Check sheet for the modelled part. Datum: model origin and axes. Units: mm. A direction names the side the tool comes from. Round coordinates to 2 decimals unless told otherwise and drop trailing zeros. Write each loop counter-clockwise with the first axis right and the second up, starting at its lowest first coordinate (ties: lowest second). Pieces come first, ordered by that corner, then holes. Notation, with made-up numbers: (30.5, -35.5) - (79.5, -35.5) arc R30 cw to (79.5, -8.5) - close; hole circle Ø3 at (83, 39.25). An arc over 180 degrees is marked (long way). Answer as a JSON object with one key per item and string values. Group by question number.
Item 1: Thickness scan on line 1 (Z direction, x = -5.25, y = 4) (3 decimals); line 2 (Y direction, x = 1.5, z = -66.5); line 3 (Y direction, x = 0.25, z = -3.5). Record the ranges inside material, lowest first.
Item 2: Sectioned sample at B-B on z = 7.5. Record the boundary of the cut face in (x, y) (3 decimals), plus the area to 3 significant figures.
Item 3: Release check for a two-part mould opening along Z. For faces 1 (the flat face through (2, -3, -53.975)), 2 (the flat face through (0.1, 3.4, 63.5)), 3 (the flat face through (5.657, -6.238, 61.89)) record: pulls with the +Z half, pulls with the -Z half, needs draft (parallel to the pull), parting line crosses it, or undercut.
Item 4: Set-up check for faces 4 (the cylindrical face through (-0.69, -3.1, -69.94)), 5 (the cylindrical face through (6.194, 0.039, 61.89)), 6 (the cylindrical face through (-3.78, -2.9, 57.43)): record each of +Z, -Z, +X, -X, +Y, -Y from which the full face is reachable in a straight line by a thin tool's end or side.
Item 5: Gauge pin test, flat ends, axial feed: P1, Ø1.5, axis at x = -2.5, y = -10.5, coming from the +Z side; P2, Ø4, axis at x = 3, z = -51.5, coming from the +Y side; P3, Ø6, axis at y = -5.5, z = -44, coming from the -X side. Record the tip position at first contact, or that the pin passes through.
```python
from build123d import *

# Parameters (mm, degrees)
SKETCH1_R           = 3.175
BOSS_EXTRUDE1_DEPTH = 53.975
SKETCH2_R           = 4.7625
BOSS_EXTRUDE2_DEPTH = 6.35
BOSS_EXTRUDE3_DEPTH = 3.175
FILLET1_R           = 0.635
BOSS_EXTRUDE4_START = 12.7
SKETCH4_R           = 3.175
BOSS_EXTRUDE4_DEPTH = 12.7


with BuildPart() as part:
    # Sketch1 → Boss-Extrude1 (new body)
    with BuildSketch(Plane.XY):
        Circle(SKETCH1_R)
    boss_extrude1 = extrude(amount=BOSS_EXTRUDE1_DEPTH)

    # Sketch2 → Boss-Extrude2 (add)
    with BuildSketch(Plane.XY.offset(53.975)):
        Circle(SKETCH2_R)
    boss_extrude2 = extrude(amount=BOSS_EXTRUDE2_DEPTH)

    # Sketch3 → Boss-Extrude3 (add)
    with BuildSketch(Plane.XY.offset(60.325)):
        with BuildLine():
            Line((-0.215682611, 14.2875), (0.215682611, 14.2875))
            ThreePointArc((0.215682611, 14.2875), (3.60364364, 12.992750331), (5.264611983, 9.768492152))
            Line((5.264611983, 9.768492152), (6.038337693, 2.804960762))
            ThreePointArc((6.038337693, 2.804960762), (6.193690832, 0), (6.038337693, -2.804960762))
            Line((6.038337693, -2.804960762), (5.264611983, -9.768492152))
            ThreePointArc((5.264611983, -9.768492152), (3.60364364, -12.992750331), (0.215682611, -14.2875))
            Line((0.215682611, -14.2875), (-0.215682611, -14.2875))
            ThreePointArc((-0.215682611, -14.2875), (-3.60364364, -12.992750331), (-5.264611983, -9.768492152))
            Line((-5.264611983, -9.768492152), (-6.038337693, -2.804960762))
            ThreePointArc((-6.038337693, -2.804960762), (-6.193690832, 0), (-6.038337693, 2.804960762))
            Line((-6.038337693, 2.804960762), (-5.264611983, 9.768492152))
            ThreePointArc((-5.264611983, 9.768492152), (-3.60364364, 12.992750331), (-0.215682611, 14.2875))
        make_face()
    boss_extrude3 = extrude(amount=BOSS_EXTRUDE3_DEPTH)

    # Mirror1: Boss-Extrude1, Boss-Extrude2, Boss-Extrude3 across plane
    add(boss_extrude1.mirror(Plane.XY))
    add(boss_extrude2.mirror(Plane.XY))
    add(boss_extrude3.mirror(Plane.XY))

    # Fillet1
    fillet1_edges = [part.edges().sort_by_distance(p)[0] for p in [
        (-4.7625, 0, -53.975),
        (-4.7625, 0, 53.975),
    ]]
    fillet(fillet1_edges, radius=FILLET1_R)

    # Sketch4 → Boss-Extrude4 (add)
    with BuildSketch(Plane.XY.offset(63.5).offset(BOSS_EXTRUDE4_START)):
        Circle(SKETCH4_R)
    boss_extrude4 = extrude(amount=-BOSS_EXTRUDE4_DEPTH)

    # Mirror2: Boss-Extrude4 across plane
    add(boss_extrude4.mirror(Plane.XY))


solid = part.part
```
Completed:
{
 "1": {"line 1": "-63.5 to -60.325, 60.325 to 63.5", "line 2": "-2.8 to 2.8", "line 3": "-3.17 to 3.17"},
 "2": {"outline": "circle Ø6.35 at (0, 0)", "area": "31.7 mm²"},
 "3": {"face 1": "undercut", "face 2": "pulls with the +Z half", "face 3": "needs draft"},
 "4": {"face 4": "-Z", "face 5": "+Z, -Z, +X", "face 6": "none"},
 "5": {"P1": "z = 63.5", "P2": "y = 3.01", "P3": "x = -1.96"}
}
